```python
from build123d import *

# Parameters (mm, degrees)
BOSS_EXTRUDE1_DEPTH = 3
CUT_EXTRUDE1_DEPTH  = 443.992475482
CIRPATTERN1_COUNT   = 3
CUT_EXTRUDE2_DEPTH  = 443.992475482


with BuildPart() as part:
    # Sketch1 → Boss-Extrude1 (new body)
    with BuildSketch(Plane.XY):
        Polygon((334.86315613, 0), (167.431578065, 290), (-167.431578065, 290), (-334.86315613, 0), (-167.431578065, -290), (167.431578065, -290), align=None)
        Polygon((57.735026919, 100), (-57.735026919, 100), (-115.470053838, 0), (-57.735026919, -100), (57.735026919, -100), (115.470053838, 0), align=None, mode=Mode.SUBTRACT)
    extrude(amount=BOSS_EXTRUDE1_DEPTH)

    # Sketch2 → Cut-Extrude1 (cut, through all)
    with BuildSketch(Plane(origin=(0, 0, 0), x_dir=(-1, 0, 0), z_dir=(0, 0, -1))):
        with BuildLine():
            Line((-51.188420258, 259.339055353), (-72.112031884, 223.098296941))
            ThreePointArc((-72.112031884, 223.098296941), (-72.844082691, 222.366246133), (-73.844082691, 222.098296941))
            Line((-73.844082691, 222.098296941), (-79.617585383, 222.098296941))
            ThreePointArc((-79.617585383, 222.098296941), (-81.349636191, 223.098296941), (-81.349636191, 225.098296941))
            Line((-81.349636191, 225.098296941), (-58.982648893, 263.839055353))
            ThreePointArc((-58.982648893, 263.839055353), (-57.768236175, 264.770907006), (-56.250598085, 264.571106161))
            Line((-56.250598085, 264.571106161), (-51.920471066, 262.071106161))
            ThreePointArc((-51.920471066, 262.071106161), (-50.988619413, 260.856693443), (-51.188420258, 259.339055353))
        make_face()
        with BuildLine():
            Line((56.250598085, 264.571106161), (51.920471066, 262.071106161))
            ThreePointArc((51.920471066, 262.071106161), (50.988619413, 260.856693443), (51.188420258, 259.339055353))
            Line((51.188420258, 259.339055353), (72.112031884, 223.098296941))
            ThreePointArc((72.112031884, 223.098296941), (72.844082691, 222.366246133), (73.844082691, 222.098296941))
            Line((73.844082691, 222.098296941), (79.617585383, 222.098296941))
            ThreePointArc((79.617585383, 222.098296941), (81.349636191, 223.098296941), (81.349636191, 225.098296941))
            Line((81.349636191, 225.098296941), (58.982648893, 263.839055353))
            ThreePointArc((58.982648893, 263.839055353), (57.768236175, 264.770907006), (56.250598085, 264.571106161))
        make_face()
    cut_extrude1 = extrude(amount=-CUT_EXTRUDE1_DEPTH, mode=Mode.SUBTRACT)

    # CirPattern1: Cut-Extrude1 ×3 about axis
    cirpattern1_axis = Axis((0, 0, 0), (0, 0, 1))
    for i in range(1, CIRPATTERN1_COUNT):
        add(cut_extrude1.rotate(cirpattern1_axis, i * 360 / CIRPATTERN1_COUNT), mode=Mode.SUBTRACT)

    # Sketch3 → Cut-Extrude2 (cut, through all)
    with BuildSketch(Plane.XY.offset(3)):
        with BuildLine():
            Line((-12.961481397, 174), (12.961481397, 174))
            ThreePointArc((12.961481397, 174), (14.999580058, 173.201398157), (15.952592488, 171.230769231))
            ThreePointArc((15.952592488, 171.230769231), (0, 154), (-15.952592488, 171.230769231))
            ThreePointArc((-15.952592488, 171.230769231), (-14.999580058, 173.201398157), (-12.961481397, 174))
        make_face()
        with BuildLine():
            Line((-157.169160957, -75.77502784), (-144.20767956, -98.22497216))
            ThreePointArc((-144.20767956, -98.22497216), (-142.497020746, -99.590716455), (-140.313899819, -99.430734967))
            ThreePointArc((-140.313899819, -99.430734967), (-133.367912183, -77), (-156.266492308, -71.800034264))
            ThreePointArc((-156.266492308, -71.800034264), (-157.496600804, -73.610681702), (-157.169160957, -75.77502784))
        make_face()
        with BuildLine():
            Line((157.169160957, -75.77502784), (144.20767956, -98.22497216))
            ThreePointArc((144.20767956, -98.22497216), (142.497020746, -99.590716455), (140.313899819, -99.430734967))
            ThreePointArc((140.313899819, -99.430734967), (133.367912183, -77), (156.266492308, -71.800034264))
            ThreePointArc((156.266492308, -71.800034264), (157.496600804, -73.610681702), (157.169160957, -75.77502784))
        make_face()
    extrude(amount=-CUT_EXTRUDE2_DEPTH, mode=Mode.SUBTRACT)


solid = part.part
```
Build history of the part. All positions in model axes, mm. A direction names the side the tool comes from. Give positions to 0.01 mm unless a question says otherwise; leave off trailing zeros. Order: outer loops, then holes, each group sorted by start corner. A loop starts at its lowest first (then second) coordinate and runs counter-clockwise, first axis right, second up. Notation, with made-up numbers: M -15,86.5 L -4,86.5 A35 ccw -4,124.5 Z; hole C 71,79.5 d10. An arc over 180 degrees is marked long. Return JSON: item names as keys, results as strings.
Q1. Band-saw the part on D-D (y = 125). Give the cut face in (x, z), then the cut area to 3 significant figures.
Answer list:
{"outline": "M -262.69,0 L 262.69,0 L 262.69,3 L -262.69,3 Z", "area": "1,580 mm^2"}
Q2. Band-saw the part on B-B (y = 23). Give the cut face in (x, z), then the cut area to 3 significant figures.
Answer list:
{"outline": "M -321.58,0 L -102.19,0 L -102.19,3 L -321.58,3 Z; M 102.19,0 L 321.58,0 L 321.58,3 L 102.19,3 Z", "area": "1,320 mm^2"}
Q3. Flat gauge pins, fed straight in: pin 1 (1.5 mm diameter, centred on y = -57.5, z = 1, fed in from -X); pin 2 (1.5 mm diameter, centred on x = 169.5, z = 1, fed in from +Y); pin 3 (5 mm diameter, centred on x = -87.5, y = 41.5, fed in from +Z); pin 4 (1 mm diameter, centred on y = -27, z = 2.5, fed in from -X). Where does each tip first touch, or does it go through?
Answer list:
{"pin 1": "stops at x = -302.1", "pin 2": "stops at y = 287.72", "pin 3": "passes through", "pin 4": "stops at x = -319.56"}
Q4. Wall check: probe 1 along Y at (x, z) = (21, 2.7); probe 2 along X at (y, z) = (-55, 2.4); probe 3 along X at (y, z) = (230, 2). Give the ranges that are in metal, low to high. Write a range as from..to.
Answer list:
{"probe 1": "y = -290..-100, 100..290", "probe 2": "x = -303.11..-243.06, -232.67..-83.72, 83.72..232.67, 243.06..303.11", "probe 3": "x = -202.07..-78.52, -68.13..68.13, 78.52..202.07"}
Q5. Two-plate mould, pull along Y, no slides. Class faces 1 (the face through (252.3, 143, 1.5)), 2 (the face through (-79, 69, 3)), 3 (the face through (0, 154, 2)): pulls with the +Y half, pulls with the -Y half, needs draft (parallel to the pull), parting line crosses it, or undercut.
Answer list:
{"face 1": "pulls with the +Y half", "face 2": "needs draft", "face 3": "undercut"}
Q6. Band-saw the part on C-C (z = 1.9). Count the separate pieces of the cut face and the enclosed holes in it, then the cut area to 3 significant figures.
Answer list:
{"separate pieces": "1", "enclosed holes": "10", "area": "253,000 mm^2"}
Q7. Band-saw the part on A-A (x = -33). Give the cut face in (y, z), then the cut area to 3 significant figures.
Answer list:
{"outline": "M -290,0 L -100,0 L -100,3 L -290,3 Z; M 100,0 L 290,0 L 290,3 L 100,3 Z", "area": "1,140 mm^2"}
Q8. 3-axis set-ups, long thin cutter, end or side, ignore diameter. For faces 4 (the face through (-246.643, -61.197, 1.479)), 5 (the face through (-252.3, -143, 1.5)): which of +Z, -Z, +X, -X, +Y, -Y reach the whole face in a straight line?
Answer list:
{"face 4": "+Z, -Z", "face 5": "+Z, -Z, -X, -Y"}
